Design review of the part built by this model. Coordinates are the model's own, in mm. A direction names the side the tool comes from. Give positions to 0.01 mm unless a question says otherwise; leave off trailing zeros. Loops run counter-clockwise (first coordinate to the right, second up) from the corner with the lowest first, then second, coordinate; pieces in that order, holes last. Notation, with made-up numbers: (36, 9) -> (78, 9) arc R9 ccw to (78, 25) -> close; hole circle Ø3 at (80.5, 32). An arc over 180 degrees is marked (long way). Answer in a Markdown table with one row per item. Add a question column.
(1) Draft analysis for pull direction Z (two halves, no side actions). For faces 1 (the flat face through (10.739, -29, -47)), 2 (the flat face through (17.239, -19, -26)), 3 (the flat face through (0, -23, 48.25)), 4 (the flat face through (15, -17, -7.486)), state which applies: +Z half, -Z half, draft (parallel to the pull), parting line (faces both ways), or undercut.
(2) Consider section C-C on z = 14.5. Write out the cut boundary in (x, y).
(3) Consider section B-B on x = 13.5. Write out the cut boundary in (y, z), then the cut area to 3 significant figures.
(4) Consider section D-D on y = -27.5. Write out the cut boundary in (x, z).
(5) For faces 5 (the flat face through (0.739, -29, -47)), 6 (the flat face through (-17, -28, -45.25)), 7 (the flat face through (15.739, -33, -47)), list the 3-axis set-ups (+Z, -Z, +X, -X, +Y, -Y) from which the entire face can be reached by the end or side of a thin tool; tool diameter is ignored.
(6) For pin 1 (1.5 mm diameter, centred on y = -32, z = -47, fed in from +X); pin 2 (3.5 mm diameter, centred on y = -30, z = 46.5, fed in from +X); pin 3 (1 mm diameter, centred on y = -17, z = 2, fed in from +X); pin 4 (1.5 mm diameter, centred on x = -6, y = -23, fed in from +Z), all flat-tipped, find the tip position at first contact; note any pin that passes through.
(7) For line 1 (Z direction, x = 12, y = -34.5); line 2 (Y direction, x = -8, z = 34.5), list the stretches that pass through material, from the lowest coordinate up.
(8) Consider section A-A on y = -33. Write out the cut boundary in (x, z).
from build123d import *

# Parameters (mm, degrees)
SKETCH8_W           = 40
SKETCH8_H           = 20
BOSS_EXTRUDE1_DEPTH = 48.25
SKETCH10_W          = 36.5
SKETCH10_H          = 90.5
CUT_EXTRUDE6_DEPTH  = 18
SKETCH12_W          = 90.5
SKETCH12_H          = 15.5
CUT_EXTRUDE9_DEPTH  = 28
CUT_EXTRUDE10_DEPTH = 97.5
SKETCH14_W          = 13
SKETCH14_H          = 14.985683259
CUT_EXTRUDE11_DEPTH = 10
FILLET6_R           = 2.5
CUT_EXTRUDE12_DEPTH = 97.5


with BuildPart() as part:
    # Sketch8 → Boss-Extrude1 (new body, symmetric)
    with BuildSketch(Plane.XY):
        with Locations((0.738550377, -25.566858374)):
            Rectangle(SKETCH8_W, SKETCH8_H)
    extrude(amount=BOSS_EXTRUDE1_DEPTH, both=True)

    # Sketch10 → Cut-Extrude6 (cut)
    with BuildSketch(Plane(origin=(0, -35.566858374, 0), x_dir=(1, 0, 0), z_dir=(0, 1, 0))):
        with Locations((-1.011449623, 0)):
            Rectangle(SKETCH10_W, SKETCH10_H)
    extrude(amount=CUT_EXTRUDE6_DEPTH, mode=Mode.SUBTRACT)

    # Sketch12 → Cut-Extrude9 (cut)
    with BuildSketch(Plane(origin=(20.738550377, 0, 0), x_dir=(0, 0, -1), z_dir=(1, 0, 0))):
        with Locations((0, -27.816858374)):
            Rectangle(SKETCH12_W, SKETCH12_H)
    extrude(amount=-CUT_EXTRUDE9_DEPTH, mode=Mode.SUBTRACT)

    # Sketch13 → Cut-Extrude10 (cut, through all)
    with BuildSketch(Plane.XY.offset(48.25)):
        with BuildLine():
            Line((15.738550377, -35.566858374), (20.738550377, -35.566858374))
            Line((20.738550377, -35.566858374), (20.738550377, -15.566858374))
            ThreePointArc((20.738550377, -15.566858374), (17.021467925, -22.661164224), (15.738550377, -30.566858374))
            Line((15.738550377, -30.566858374), (15.738550377, -35.566858374))
        make_face()
    extrude(amount=-CUT_EXTRUDE10_DEPTH, mode=Mode.SUBTRACT)

    # Sketch14 → Cut-Extrude11 (cut)
    with BuildSketch(Plane.XZ.offset(15.566858374)):
        with Locations((15.738550377, 0.007158371)):
            Rectangle(SKETCH14_W, SKETCH14_H)
    extrude(amount=CUT_EXTRUDE11_DEPTH, mode=Mode.SUBTRACT)

    # Fillet6
    fillet6_edges = [part.edges().sort_by_distance(p)[0] for p in [
        (-1.011449623, -17.566858374, 45.25),
        (-1.011449623, -17.566858374, -45.25),
    ]]
    fillet(fillet6_edges, radius=FILLET6_R)

    # Sketch15 → Cut-Extrude12 (cut, through all)
    with BuildSketch(Plane.XY.offset(48.25)):
        with BuildLine():
            Line((-14.261449623, -35.566858374), (-4.261449623, -35.566858374))
            Line((-4.261449623, -35.566858374), (-4.261449623, -23.066858374))
            ThreePointArc((-4.261449623, -23.066858374), (-9.261449623, -18.066858374), (-14.261449623, -23.066858374))
            Line((-14.261449623, -23.066858374), (-14.261449623, -35.566858374))
        make_face()
        with BuildLine():
            Line((10.738550377, -35.566858374), (0.738550377, -35.566858374))
            Line((0.738550377, -35.566858374), (0.738550377, -23.066858374))
            ThreePointArc((0.738550377, -23.066858374), (5.738550377, -18.066858374), (10.738550377, -23.066858374))
            Line((10.738550377, -23.066858374), (10.738550377, -35.566858374))
        make_face()
    extrude(amount=-CUT_EXTRUDE12_DEPTH, mode=Mode.SUBTRACT)


solid = part.part
Values follow:
| question | item | result |
|---|---|---|
| 1 | face 1 | draft |
| 1 | face 2 | undercut |
| 1 | face 3 | +Z half |
| 1 | face 4 | undercut |
| 2 | outline | (-19.26, -17.57) -> (17.24, -17.57) -> (17.24, -20.07) -> (18.05, -20.07) arc R25 cw to (20.74, -15.57) -> (-19.26, -15.57) -> close |
| 3 | outline | (-35.57, -48.25) -> (-15.57, -48.25) -> (-15.57, -7.49) -> (-17.57, -7.49) -> (-17.57, -42.75) arc R2.5 cw to (-20.07, -45.25) -> (-35.57, -45.25) -> close; (-35.57, 45.25) -> (-20.07, 45.25) arc R2.5 cw to (-17.57, 42.75) -> (-17.57, 7.5) -> (-15.57, 7.5) -> (-15.57, 48.25) -> (-35.57, 48.25) -> close |
| 3 | area | 274 mm2 |
| 4 | outline | (-19.26, -48.25) -> (-14.26, -48.25) -> (-14.26, -45.25) -> (-19.26, -45.25) -> close; (-19.26, 45.25) -> (-14.26, 45.25) -> (-14.26, 48.25) -> (-19.26, 48.25) -> close; (-4.26, -48.25) -> (0.74, -48.25) -> (0.74, -45.25) -> (-4.26, -45.25) -> close; (-4.26, 45.25) -> (0.74, 45.25) -> (0.74, 48.25) -> (-4.26, 48.25) -> close; (10.74, -48.25) -> (15.93, -48.25) -> (15.93, -45.25) -> (10.74, -45.25) -> close; (10.74, 45.25) -> (15.93, 45.25) -> (15.93, 48.25) -> (10.74, 48.25) -> close |
| 5 | face 5 | +Z, -Z, -Y |
| 5 | face 6 | +X, -X, -Y |
| 5 | face 7 | +Z, -Z, +X, -Y |
| 6 | pin 1 | x = 15.74 |
| 6 | pin 2 | x = 15.85 |
| 6 | pin 3 | x = 9.24 |
| 6 | pin 4 | through |
| 7 | line 1 | -48.25 to -45.25, 45.25 to 48.25 |
| 7 | line 2 | -17.57 to -15.57 |
| 8 | outline | (-19.26, -48.25) -> (-14.26, -48.25) -> (-14.26, -45.25) -> (-19.26, -45.25) -> close; (-19.26, 45.25) -> (-14.26, 45.25) -> (-14.26, 48.25) -> (-19.26, 48.25) -> close; (-4.26, -48.25) -> (0.74, -48.25) -> (0.74, -45.25) -> (-4.26, -45.25) -> close; (-4.26, 45.25) -> (0.74, 45.25) -> (0.74, 48.25) -> (-4.26, 48.25) -> close; (10.74, -48.25) -> (15.74, -48.25) -> (15.74, -45.25) -> (10.74, -45.25) -> close; (10.74, 45.25) -> (15.74, 45.25) -> (15.74, 48.25) -> (10.74, 48.25) -> close |
